CAD build for the part. Positions are in the model's coordinates, mm. A direction names the side the tool comes from. Coordinates: 2 decimals unless noted, no trailing zeros. Write each loop counter-clockwise with the first axis right and the second up, starting at its lowest first coordinate (ties: lowest second). Pieces come first, ordered by that corner, then holes.
```python
from build123d import *

# Parameters (mm, degrees)
SKETCH1_R           = 3.175
BOSS_EXTRUDE1_DEPTH = 4.7625
SKETCH3_W           = 4.7625
SKETCH3_H           = 33.783
SKETCH3_H_2         = 46.289475607
CUT_EXTRUDE2_DEPTH  = 10


with BuildPart() as part:
    # Sketch1 → Boss-Extrude1 (new body)
    with BuildSketch(Plane(origin=(0, 0, 0), x_dir=(1, 0, 0), z_dir=(0, 1, 0))):
        with BuildLine():
            Line((0, 0), (-83.629476528, 83.629476528))
            ThreePointArc((-83.629476528, 83.629476528), (-85.081850373, 100.91197572), (-70.310188895, 110))
            Line((-70.310188895, 110), (-56.601944845, 110))
            Line((-56.601944845, 110), (0, 94.833554589))
            Line((0, 94.833554589), (0, 58.293))
            Line((0, 58.293), (8, 58.293))
            Line((8, 58.293), (8, -58.293))
            Line((8, -58.293), (0, -58.293))
            Line((0, -58.293), (0, -94.833554589))
            Line((0, -94.833554589), (-56.601944845, -110))
            Line((-56.601944845, -110), (-70.310188895, -110))
            ThreePointArc((-70.310188895, -110), (-85.081850373, -100.91197572), (-83.629476528, -83.629476528))
            Line((-83.629476528, -83.629476528), (0, 0))
        make_face()
        with Locations((-70.310188895, 93.451069294)):
            Circle(SKETCH1_R, mode=Mode.SUBTRACT)
        with Locations((-70.310188895, -93.451069294)):
            Circle(SKETCH1_R, mode=Mode.SUBTRACT)
    extrude(amount=BOSS_EXTRUDE1_DEPTH)

    # Sketch3 → Cut-Extrude2 (cut)
    with BuildSketch(Plane(origin=(0, 0, 0), x_dir=(1, 0, 0), z_dir=(0, 1, 0))):
        Polygon((-4.829629131, 96.127649814), (-17.19282542, 99.440358276), (-18.425451123, 94.840136528), (-6.062254834, 91.527428067), align=None)
        Polygon((-24.920232031, 101.510910637), (-37.283428319, 104.823619098), (-38.516054022, 100.22339735), (-26.152857733, 96.910688889), align=None)
        with Locations((5.61875, 33.4015)):
            Rectangle(SKETCH3_W, SKETCH3_H)
        Polygon((-26.152857733, -96.910688889), (-38.516054022, -100.22339735), (-37.283428319, -104.823619098), (-24.920232031, -101.510910637), align=None)
        Polygon((-6.062254834, -91.527428067), (-18.425451123, -94.840136528), (-17.19282542, -99.440358276), (-4.829629131, -96.127649814), align=None)
        with Locations((5.61875, -39.654737804)):
            Rectangle(SKETCH3_W, SKETCH3_H_2)
    extrude(amount=CUT_EXTRUDE2_DEPTH, mode=Mode.SUBTRACT)


solid = part.part
```
Item 1: Flat gauge pins, fed straight in: pin 1 Ø1.4 at (x, y) = (6.5, 3) entering from +Z; pin 2 Ø1.4 at (y, z) = (3.5, 81.5) entering from +X; pin 3 Ø4 at (x, z) = (-70.31, -93.45) entering from +Y. Where does each tip first touch, or does it go through?
Item 2: Wall check: line 1 along Z through (x, y) = (4, 3.7); line 2 along Z through (x, y) = (-57, 3.85); line 3 along X through (y, z) = (1.6, 13). Give the ranges that are in metal, low to high.
Item 3: Saw through at D-D, the plane y = 0.95. State how many separate pieces and enclosed holes the cut face has, and give its area (3 significant figures).
Item 4: Saw through at B-B, the plane z = -30.5. Write the cut outline in (x, y), and give its area (3 significant figures).
Item 5: Which spindle directions (+Z, -Z, +X, -X, +Y, -Y) get a long thin tool onto all of the face, cutting with end or side? Do faces 1 (the flat face through (-37.89, 2.35, -102.56)), 2 (the flat face through (0, 2, -77)), 3 (the flat face through (-41, 2, -41)), 4 (the flat face through (-5.455, 2.348, -93.795)). Say none if no direction does.
Item 6: Saw through at C-C, the plane x = -78.5. Write the cut outline in (y, z).
Item 7: Two-plate mould, pull along X, no slides. Class faces 5 (the flat face through (-63, 2, 110)), 6 (the flat face through (-12.3, 2.3, -93.2)), 7 (the flat face through (-42, 2, 42)): +X half, -X half, draft (parallel to the pull), parting line (faces both ways), or undercut.
Item 8: Saw through at A-A, the plane x = -42.5. Write the cut outline in (y, z), and give its area (3 significant figures).
Working result:
1. pin 1: stops at z = 16.51
1. pin 2: stops at x = 0
1. pin 3: passes through
2. line 1: z = -58.29 to -50.29, -16.51 to 16.51
2. line 2: z = -110 to -57, 57 to 110
2. line 3: x = -13 to 8
3. separate pieces: 1
3. enclosed holes: 2
3. area: 10,800 mm2
4. outline: (-30.5, 0) - (3.24, 0) - (3.24, 4.76) - (-30.5, 4.76) - close
4. area: 161 mm2
5. face 1: +Y, -Y
5. face 2: -Z, +X, +Y, -Y
5. face 3: -X, +Y, -Y
5. face 4: -Z, +Y, -Y
6. outline: (0, -107.83) - (4.76, -107.83) - (4.76, -78.5) - (0, -78.5) - close; (0, 78.5) - (4.76, 78.5) - (4.76, 107.83) - (0, 107.83) - close
7. face 5: draft
7. face 6: undercut
7. face 7: -X half
8. outline: (0, -106.22) - (4.76, -106.22) - (4.76, -42.5) - (0, -42.5) - close; (0, 42.5) - (4.76, 42.5) - (4.76, 106.22) - (0, 106.22) - close
8. area: 607 mm2
